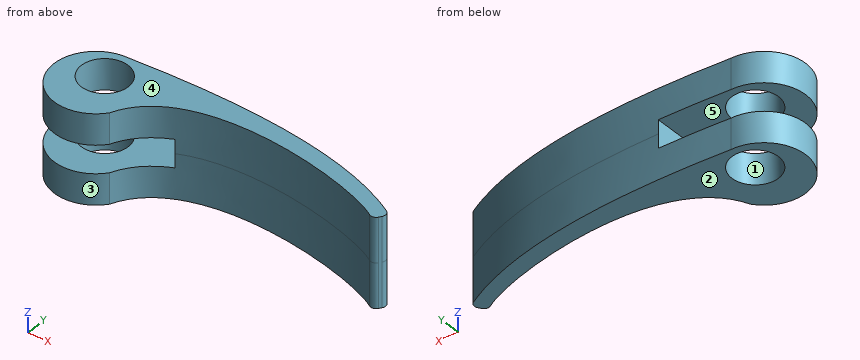
from build123d import *

# Parameters (mm, degrees)
SKETCH_R          = 4.2
PAD_DEPTH         = 8
FILLET_R          = 1
SKETCH001_W       = 28.61805
SKETCH001_H       = 5
POCKET_DEPTH      = 6.359373
POCKET_DEPTH_BACK = -9.501


with BuildPart() as part:
    # Sketch → Pad (new body, symmetric)
    with BuildSketch(Plane.XY):
        with BuildLine():
            ThreePointArc((0, 5.5), (-6.69683, -5.376754), (6.030279, -6.459343))
            add(Edge.make_bspline(
                [(6.030279, -6.459343), (11.977673, 9.279221), (47.159592, 0.679194), (50.755966, -3.073543)],
                knots=[0, 0, 0, 0, 1, 1, 1, 1], degree=3))
            Line((50.755966, -3.073543), (52.204102, -0.7977))
            add(Edge.make_bspline(
                [(0, 5.5), (35.91824, 8.824372), (52.204102, -0.7977)],
                knots=[0, 0, 0, 1, 1, 1], degree=2, weights=[8, 8, 7.92]))
        make_face()
        Circle(SKETCH_R, mode=Mode.SUBTRACT)
    extrude(amount=PAD_DEPTH, both=True)

    # Fillet
    fillet_edges = [part.edges().sort_by_distance(p)[0] for p in [
        (50.755966, -3.073543, 0),
        (52.204102, -0.7977, 0),
    ]]
    fillet(fillet_edges, radius=FILLET_R)

    # Sketch001 → Pocket (cut, two sides)
    with BuildSketch(Plane.XZ) as pocket_sk:
        with Locations((-1.773529, 0)):
            Rectangle(SKETCH001_W, SKETCH001_H)
    extrude(amount=-POCKET_DEPTH, mode=Mode.SUBTRACT)
    extrude(pocket_sk.sketch, amount=-POCKET_DEPTH_BACK, mode=Mode.SUBTRACT)


solid = part.part
Geometry check sheet. Reference: the model listing, model coordinates, mm. Face numbers are marked on the shaded views. A direction names the side the tool comes from. Give positions to 0.01 mm unless a question says otherwise; leave off trailing zeros. Answer as a JSON object with one key per item and string values. Group by question number.
Item 1: Access from +Z, -Z, +X, -X, +Y, -Y to the whole of each face (thin tool, end or side, straight path). Record for the marked faces 4 and 5.
Item 2: Sectioned sample at A-A on y = -1. Give the number of separate pieces and of enclosed holes in the cut face, plus the area to 3 significant figures.
Item 3: Mould release check, pull along Y, two halves, no side actions. Record for the marked faces 1, 2 and 3: pulls with the +Y half, pulls with the -Y half, needs draft (parallel to the pull), parting line crosses it, or undercut.
Item 4: Material ranges on L1, parallel to X at y = -3.25, z = -3; L2, parallel to X at y = -2.75, z = 3.5; L3, parallel to Y at x = -1.5, z = 6.75, recorded low to high.
Item 5: Gauge pin test, flat ends, axial feed: pin 1 (4 mm diameter, centred on y = 2, z = -1, fed in from -X); pin 2 (2 mm diameter, centred on y = 2.5, z = -3, fed in from -X); pin 3 (5 mm diameter, centred on x = 37.5, z = -2, fed in from -Y). Record the tip position at first contact, or that the pin passes through.
Findings below:
{
 "1": {"face 4": "+Z, +X, -X, +Y, -Y", "face 5": "-X, +Y, -Y"},
 "2": {"separate pieces": "5", "enclosed holes": "0", "area": "186 mm2"},
 "3": {"face 1": "undercut", "face 2": "needs draft", "face 3": "parting line crosses it"},
 "4": {"L1": "-7.4 to -2.66, 2.66 to 7.89", "L2": "-7.46 to -3.17, 3.17 to 8.33", "L3": "-9.35 to -3.92, 3.92 to 5.35"},
 "5": {"pin 1": "x = -7.01", "pin 2": "x = -6.63", "pin 3": "y = 0.97"}
}
